```python
from build123d import *

# Parameters (mm, degrees)
RESSALTO_EXTRUS_O4_DEPTH = 3
CORTE_EXTRUS_O1_DEPTH    = 3


with BuildPart() as part:
    # Esboço2 → Ressalto-extrusão4 (new body)
    with BuildSketch(Plane.XY):
        with BuildLine():
            Line((31.427362324, 25.061276238), (22.653821271, 17.699401176))
            Line((22.653821271, 17.699401176), (12.921770463, 17.699401176))
            ThreePointArc((12.921770463, 17.699401176), (12.662951418, 17.665327003), (12.421770463, 17.56542658))
            Line((12.421770463, 17.56542658), (8.55574506, 15.333375773))
            ThreePointArc((8.55574506, 15.333375773), (8.314564105, 15.23347535), (8.05574506, 15.199401176))
            Line((8.05574506, 15.199401176), (5, 15.199401176))
            ThreePointArc((5, 15.199401176), (1.464466094, 13.734935082), (0, 10.199401176))
            Line((0, 10.199401176), (0, -24.800598824))
            ThreePointArc((0, -24.800598824), (1.464466094, -28.33613273), (5, -29.800598824))
            Line((5, -29.800598824), (8.051923789, -29.800598824))
            ThreePointArc((8.051923789, -29.800598824), (8.310742834, -29.834672997), (8.551923789, -29.93457342))
            Line((8.551923789, -29.93457342), (12.587284274, -32.264389882))
            ThreePointArc((12.587284274, -32.264389882), (12.651697156, -32.298511057), (12.718424432, -32.327849506))
            ThreePointArc((12.718424432, -32.327849506), (20.804137446, -34.299176341), (29.120634875, -33.981757168))
            ThreePointArc((29.120634875, -33.981757168), (33.209608572, -35.069970557), (35, -38.903821469))
            Line((35, -38.903821469), (35, -52.300598824))
            ThreePointArc((35, -52.300598824), (33.535533906, -55.83613273), (30, -57.300598824))
            Line((30, -57.300598824), (-40, -57.300598824))
            ThreePointArc((-40, -57.300598824), (-43.535533906, -55.83613273), (-45, -52.300598824))
            Line((-45, -52.300598824), (-45, -38.903821469))
            ThreePointArc((-45, -38.903821469), (-43.209608572, -35.069970557), (-39.120634875, -33.981757168))
            ThreePointArc((-39.120634875, -33.981757168), (-30.804137446, -34.299176341), (-22.718424432, -32.327849506))
            ThreePointArc((-22.718424432, -32.327849506), (-22.651697156, -32.298511057), (-22.587284274, -32.264389882))
            Line((-22.587284274, -32.264389882), (-18.551923789, -29.93457342))
            ThreePointArc((-18.551923789, -29.93457342), (-18.310742834, -29.834672997), (-18.051923789, -29.800598824))
            Line((-18.051923789, -29.800598824), (-15, -29.800598824))
            ThreePointArc((-15, -29.800598824), (-11.464466094, -28.33613273), (-10, -24.800598824))
            Line((-10, -24.800598824), (-10, 10.199401176))
            ThreePointArc((-10, 10.199401176), (-11.464466094, 13.734935082), (-15, 15.199401176))
            Line((-15, 15.199401176), (-18.05574506, 15.199401176))
            ThreePointArc((-18.05574506, 15.199401176), (-18.314564105, 15.23347535), (-18.55574506, 15.333375773))
            Line((-18.55574506, 15.333375773), (-22.421770463, 17.56542658))
            ThreePointArc((-22.421770463, 17.56542658), (-22.662951418, 17.665327003), (-22.921770463, 17.699401176))
            Line((-22.921770463, 17.699401176), (-32.653821271, 17.699401176))
            Line((-32.653821271, 17.699401176), (-41.427362324, 25.061276238))
            ThreePointArc((-41.427362324, 25.061276238), (-44.062564097, 28.495538052), (-44.999486227, 32.721720669))
            Line((-44.999486227, 32.721720669), (-44.999486227, 77.699401176))
            Line((-44.999486227, 77.699401176), (-44.999486227, 79.699401176))
            ThreePointArc((-44.999486227, 79.699401176), (-44.12080657, 81.82072152), (-41.999486227, 82.699401176))
            Line((-41.999486227, 82.699401176), (-39.999486227, 82.699401176))
            Line((-39.999486227, 82.699401176), (29.999486227, 82.699401176))
            Line((29.999486227, 82.699401176), (31.999486227, 82.699401176))
            ThreePointArc((31.999486227, 82.699401176), (34.12080657, 81.82072152), (34.999486227, 79.699401176))
            Line((34.999486227, 79.699401176), (34.999486227, 77.699401176))
            Line((34.999486227, 77.699401176), (34.999486227, 32.721720669))
            ThreePointArc((34.999486227, 32.721720669), (34.062564097, 28.495538052), (31.427362324, 25.061276238))
        make_face()
    extrude(amount=RESSALTO_EXTRUS_O4_DEPTH)

    # Esboço3 → Corte-extrusão1 (cut)
    with BuildSketch(Plane(origin=(0, 0, 0), x_dir=(-1, 0, 0), z_dir=(0, 0, -1))):
        with BuildLine():
            Line((4.7, 15.199401176), (5.3, 15.199401176))
            ThreePointArc((5.3, 15.199401176), (6.148528137, 14.847929314), (6.5, 13.999401176))
            Line((6.5, 13.999401176), (6.5, -23.050598824))
            ThreePointArc((6.5, -23.050598824), (6.148528137, -23.899126961), (5.3, -24.250598824))
            Line((5.3, -24.250598824), (4.7, -24.250598824))
            ThreePointArc((4.7, -24.250598824), (3.851471863, -23.899126961), (3.5, -23.050598824))
            Line((3.5, -23.050598824), (3.5, 13.999401176))
            ThreePointArc((3.5, 13.999401176), (3.851471863, 14.847929314), (4.7, 15.199401176))
        make_face()
    extrude(amount=-CORTE_EXTRUS_O1_DEPTH, mode=Mode.SUBTRACT)


solid = part.part
```
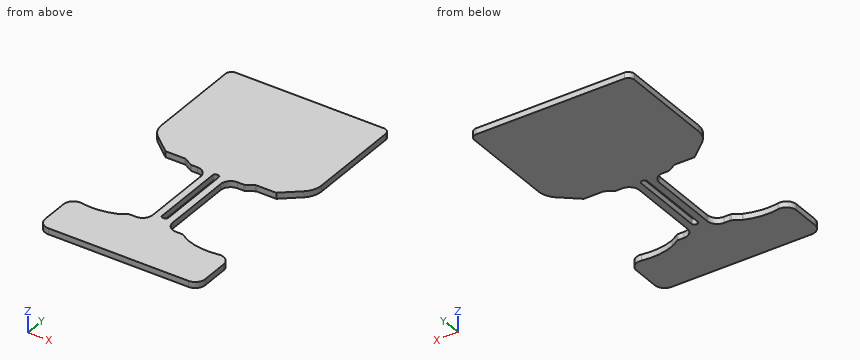
Part model, mm, in its own coordinate system. Round coordinates to 2 decimals unless told otherwise and drop trailing zeros. Loops run counter-clockwise (first coordinate to the right, second up) from the corner with the lowest first, then second, coordinate; pieces in that order, holes last. Notation, with made-up numbers: (86, 44) -> (126, 44) arc R20 ccw to (126, 64) -> close; hole circle Ø9 at (6, -17). An arc over 180 degrees is marked (long way). Use one line per item in the form item = value. Start each with the question number.
Item 1: Drill centre lines: line 1 along Y through (x, z) = (-4.5, 2.3); line 2 along X through (y, z) = (-14.5, 2); line 3 along Y through (x, z) = (7.5, 0.5). Where is each one in solid material? Low to high.
Item 2: Band-saw the part on A-A (x = -29.5). List the corners of the cut face in (y, z).
Item 3: Drop flat-ended pins along their axis: pin 1 Ø0.9 at (y, z) = (-2.5, 1.5) entering from +X; pin 2 Ø0.9 at (y, z) = (-6, 1.5) entering from -X. Give the stop position or say it passes through.
Data:
q1.line_1 = -57.3 to -24.23, 15.18 to 82.7
q1.line_2 = -10 to -6.5, -3.5 to 0
q1.line_3 = -57.3 to -29.8, 15.2 to 82.7
q2.outline = (-57.3, 0) -> (-34.14, 0) -> (-34.14, 3) -> (-57.3, 3) -> close; (17.7, 0) -> (82.7, 0) -> (82.7, 3) -> (17.7, 3) -> close
q3.pin_1 = 0
q3.pin_2 = -10
